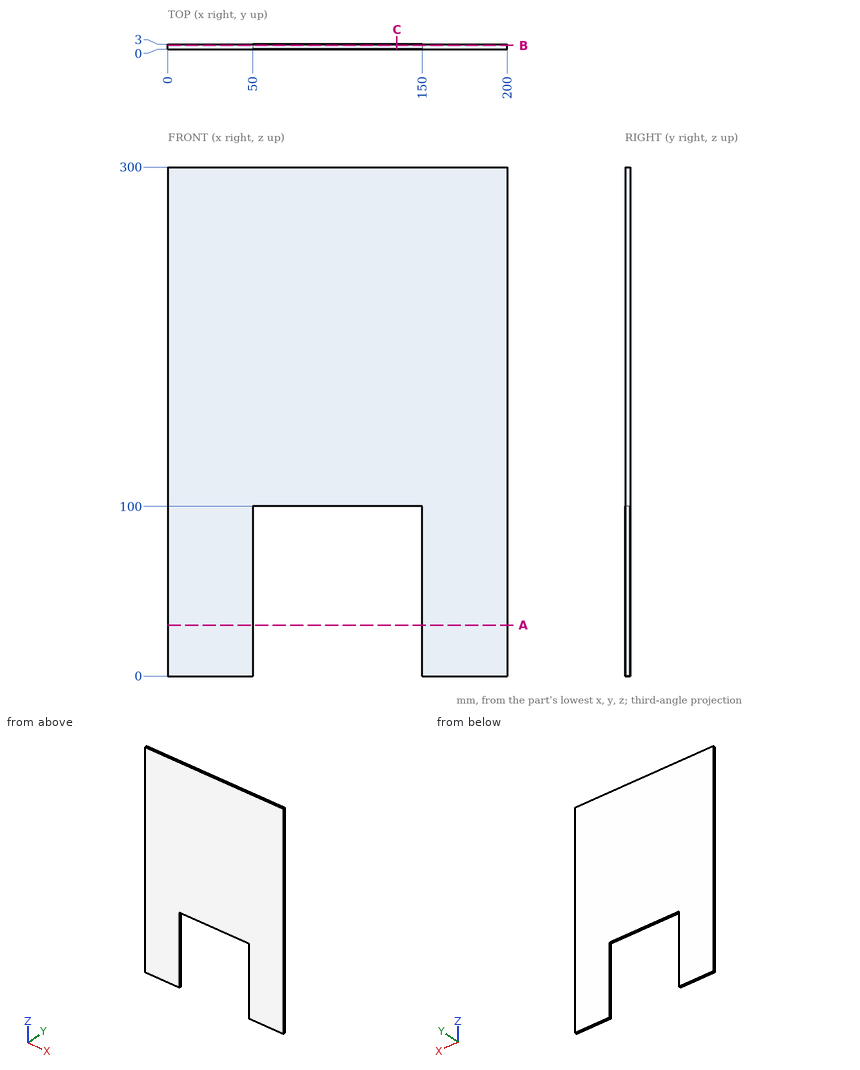
Geometry check sheet. Reference: drawing and pictorial views, mm from the part's lowest x, y, z. Round coordinates to 2 decimals unless told otherwise and drop trailing zeros. Order: outer loops, then holes, each group sorted by start corner. A loop starts at its lowest first (then second) coordinate and runs counter-clockwise, first axis right, second up. Notation, with made-up numbers: (41.5, -6.75) - (65.5, -6.75) arc R18 cw to (65.5, 21.25) - close; hole circle Ø9 at (-33.75, 59.25). An arc over 180 degrees is marked (long way). One line per question, with ' | ' between items. Start each with the question number.
(1) Depth check by flat-ended pin: pin 1 Ø1.5 at (x, y) = (123, 1.5) entering from -Z; pin 2 Ø1.5 at (y, z) = (1.5, 48.5) entering from -X. Enter the tip coordinate at first touch or a pass-through.
(2) Sectioned sample at C-C on x = 135. Record the cut outline in (y, z), and give its area (3 significant figures).
(3) Sectioned sample at B-B on y = 2.15. Record the cut outline in (x, z).
(4) Sectioned sample at A-A on z = 30. Record the cut outline in (x, y), and give its area (3 significant figures).
(5) Thickness scan on L1, parallel to X at y = 2.7, z = 47.5; L2, parallel to Z at x = 54, y = 0.6. Record the ranges inside material, lowest first. Write a range as [from, to].
Conclusion:
1) pin 1: stops at z = 100 | pin 2: stops at x = 0
2) outline: (0, 100) - (3, 100) - (3, 300) - (0, 300) - close | area: 600 mm2
3) outline: (0, 0) - (50, 0) - (50, 100) - (150, 100) - (150, 0) - (200, 0) - (200, 300) - (0, 300) - close
4) outline: (0, 0) - (50, 0) - (50, 3) - (0, 3) - close; (150, 0) - (200, 0) - (200, 3) - (150, 3) - close | area: 300 mm2
5) L1: x = [0, 50], [150, 200] | L2: z = [100, 300]
